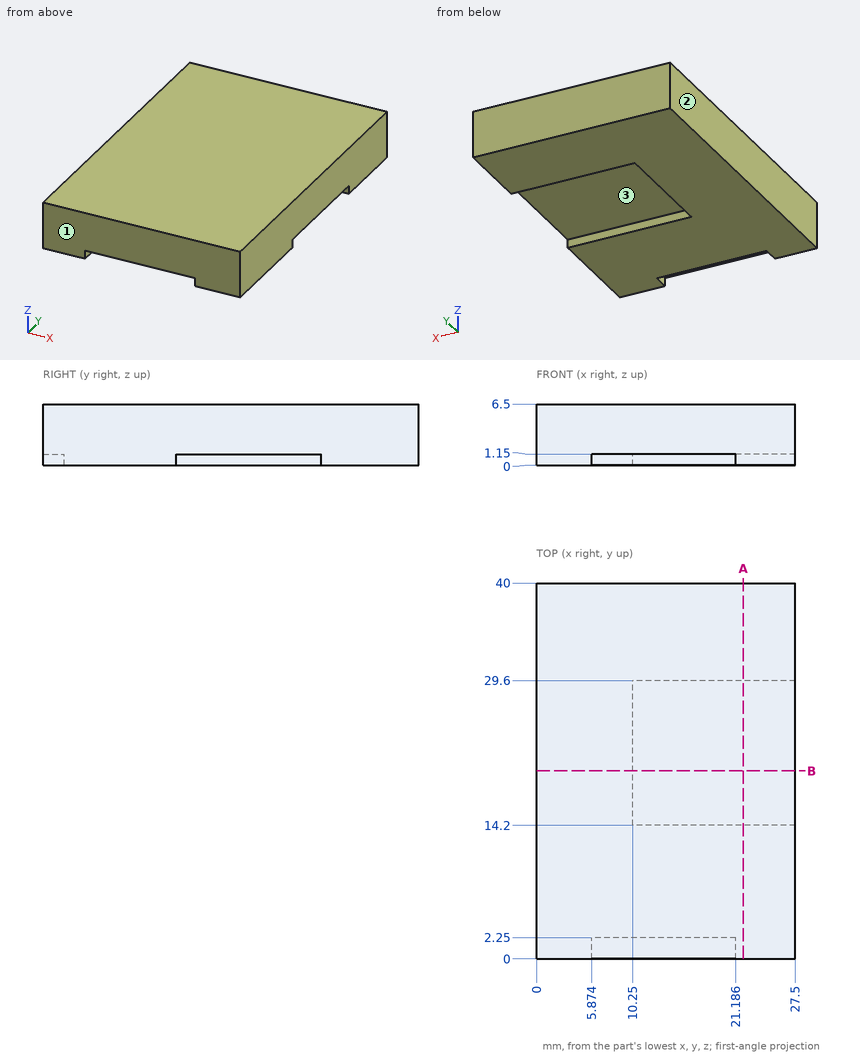
Answer from the drawing. Dimensions are ordinates in mm from the lowest x, y and z of the part. Give positions to 0.01 mm unless a question says otherwise; leave off trailing zeros. Loops run counter-clockwise (first coordinate to the right, second up) from the corner with the lowest first, then second, coordinate; pieces in that order, holes last. Notation, with made-up numbers: (-40, 3) - (-1, 3) arc R20 ccw to (-1, 12) - close; hole circle Ø11 at (-1, -38.5). An arc over 180 degrees is marked (long way). Answer as CSV lines item,"result". Start each with the question number.
Item 1: Find the intervals of material crossed by line 1 (Y direction, x = 14, z = 1); line 2 (X direction, y = 17, z = 0.5); line 3 (Z direction, x = 21.5, y = 24), in increasing order. Write a range as from..to.
Item 2: Each of these flat-tipped pins is pushed along its axis until it touches: pin 1 (7.5 mm diameter, centred on x = 16.5, y = 23.5, fed in from -Z); pin 2 (0.6 mm diameter, centred on x = 15.5, z = 0.5, fed in from -Y); pin 3 (0.6 mm diameter, centred on y = 23, z = 0.5, fed in from +X). Where does it stop, or does it pass through?
Item 3: A cutting plane is placed at B-B on y = 20. Determine the outline of the cut face in (x, z), then the cut area to 3 significant figures.
Item 4: The mould has two halves that part along Y. Classify the marked faces 1, 2 and 3: +Y half, -Y half, draft (parallel to the pull), parting line (faces both ways), or undercut.
Item 5: A cutting plane is placed at A-A on x = 22. Determine the outline of the cut face in (y, z), then the cut area to 3 significant figures.
Found:
1,line 1,"y = 2.25..14.2, 29.6..40"
1,line 2,"x = 0..10.25"
1,line 3,"z = 1.15..6.5"
2,pin 1,"stops at z = 1.15"
2,pin 2,"stops at y = 2.25"
2,pin 3,"stops at x = 10.25"
3,outline,"(0, 0) - (10.25, 0) - (10.25, 1.15) - (27.5, 1.15) - (27.5, 6.5) - (0, 6.5) - close"
3,area,"159 mm^2"
4,face 1,"-Y half"
4,face 2,"draft"
4,face 3,"undercut"
5,outline,"(0, 0) - (14.2, 0) - (14.2, 1.15) - (29.6, 1.15) - (29.6, 0) - (40, 0) - (40, 6.5) - (0, 6.5) - close"
5,area,"242 mm^2"
